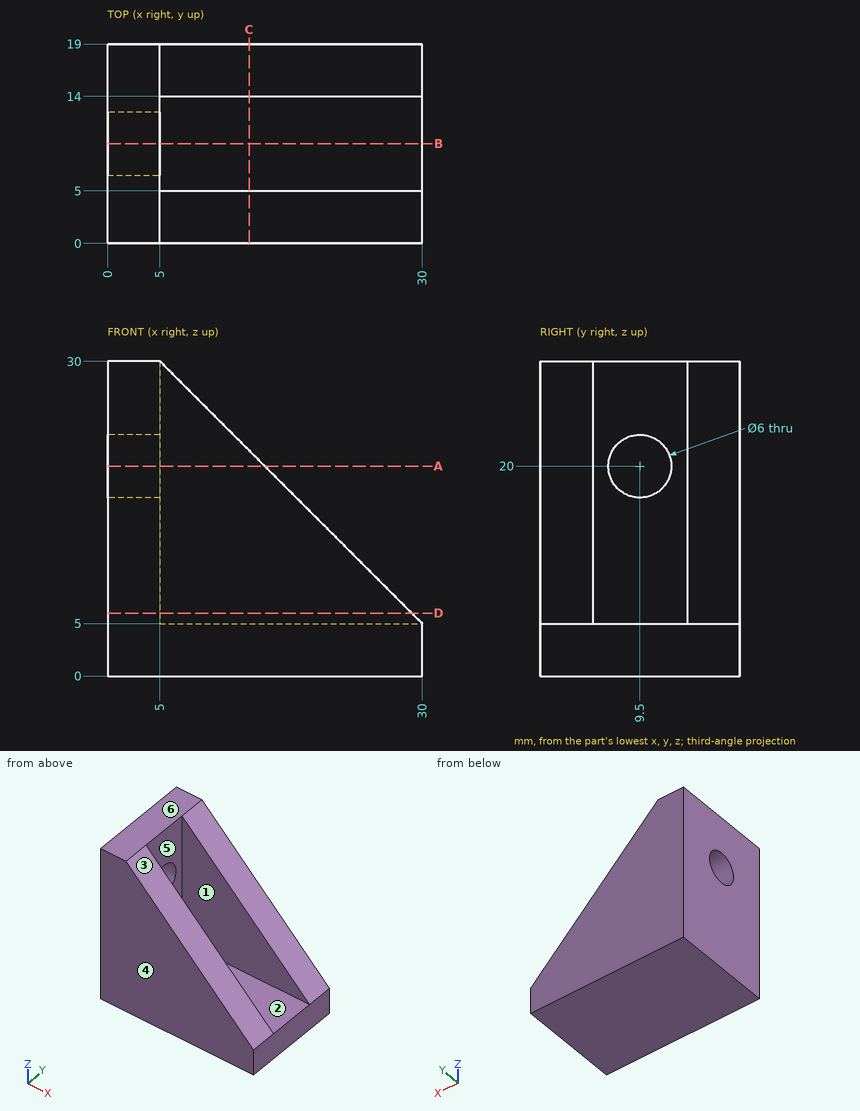
Geometry check sheet. Reference: drawing and pictorial views, mm from the part's lowest x, y, z. A direction names the side the tool comes from. Round coordinates to 2 decimals unless told otherwise and drop trailing zeros. Loops run counter-clockwise (first coordinate to the right, second up) from the corner with the lowest first, then second, coordinate; pieces in that order, holes last. Notation, with made-up numbers: (-12.75, 14.25) -> (-2.75, 14.25) arc R7 ccw to (-2.75, 18.25) -> close; hole circle Ø6 at (23, 30.5). An arc over 180 degrees is marked (long way). Answer as a JSON object with one key per item and string values. Group by question number.
Item 1: Thickness scan on line 1 along Z through (x, y) = (3.1, 9.5); line 2 along Z through (x, y) = (26, 8.75). Record the ranges inside material, lowest first.
Item 2: Cross-section at B-B, the plane y = 9.5. Record the cut outline in (x, z).
Item 3: Cross-section at D-D, the plane z = 6. Record the cut outline in (x, y), plus the area to 3 significant figures.
Item 4: Set-up check for the marked faces 5 and 6: record each of +Z, -Z, +X, -X, +Y, -Y from which the full face is reachable in a straight line by a thin tool's end or side.
Item 5: Depth check by flat-ended pin: pin 1 Ø7.5 at (x, z) = (19, 17.5) entering from -Y; pin 2 Ø7 at (x, y) = (13.5, 10) entering from +Z; pin 3 Ø2 at (y, z) = (4.5, 26) entering from +X; pin 4 Ø7 at (y, z) = (8, 21) entering from +X. Enter the tip coordinate at first touch or a pass-through.
Item 6: Cross-section at C-C, the plane x = 13.5. Record the cut outline in (y, z), plus the area to 3 significant figures.
Item 7: Cross-section at A-A, the plane z = 20. Record the cut outline in (x, y).
Item 8: Release check for a two-part mould opening along Y. For the marked faces 1, 2, 3 and 4 record: pulls with the +Y half, pulls with the -Y half, needs draft (parallel to the pull), parting line crosses it, or undercut.
Determined:
{
 "1": {"line 1": "z = 0 to 17, 23 to 30", "line 2": "z = 0 to 5"},
 "2": {"outline": "(0, 0) -> (30, 0) -> (30, 5) -> (5, 5) -> (5, 17) -> (0, 17) -> close; (0, 23) -> (5, 23) -> (5, 30) -> (0, 30) -> close"},
 "3": {"outline": "(0, 0) -> (29, 0) -> (29, 5) -> (5, 5) -> (5, 14) -> (29, 14) -> (29, 19) -> (0, 19) -> close", "area": "335 mm²"},
 "4": {"face 5": "+Z, +X", "face 6": "+Z, +X, -X, +Y, -Y"},
 "5": {"pin 1": "stops at y = 0", "pin 2": "stops at z = 5", "pin 3": "stops at x = 10", "pin 4": "stops at x = 15.8"},
 "6": {"outline": "(0, 0) -> (19, 0) -> (19, 21.5) -> (14, 21.5) -> (14, 5) -> (5, 5) -> (5, 21.5) -> (0, 21.5) -> close", "area": "260 mm²"},
 "7": {"outline": "(0, 0) -> (15, 0) -> (15, 5) -> (5, 5) -> (5, 6.5) -> (0, 6.5) -> close; (0, 12.5) -> (5, 12.5) -> (5, 14) -> (15, 14) -> (15, 19) -> (0, 19) -> close"},
 "8": {"face 1": "undercut", "face 2": "undercut", "face 3": "needs draft", "face 4": "pulls with the -Y half"}
}
